from build123d import *

# Parameters (mm, degrees)
F0_W     = 99.991299
F0_H     = 51.749203
F1_DEPTH = 1
F2_R     = 3.884772
F3_DEPTH = 1.001
F4_R     = 2.651648
F5_DEPTH = 25.4


with BuildPart() as f1:
    # F0 (on Top) → F1 (new body)
    with BuildSketch(Plane.XY):
        with Locations((49.995649, 25.874601)):
            Rectangle(F0_W, F0_H)
    extrude(amount=F1_DEPTH)

    # F2 (on face) → F3 (cut, through all)
    with BuildSketch(Plane.XY.offset(1)):
        with Locations((73.43898, 21.35068)):
            Circle(F2_R)
    extrude(amount=-F3_DEPTH, mode=Mode.SUBTRACT)

    # F4 (on face) → F5 (join)
    with BuildSketch(Plane.XY.offset(1)):
        with Locations((28.457584, 20.000773)):
            Circle(F4_R)
    extrude(amount=F5_DEPTH)


solid = f1.part
Can you work these out from the model? Positions are in its coordinate system, mm. Coordinates: 2 decimals unless noted, no trailing zeros. Write each loop counter-clockwise with the first axis right and the second up, starting at its lowest first coordinate (ties: lowest second). Pieces come first, ordered by that corner, then holes. Notation, with made-up numbers: (39.5, 79.25) - (97.5, 79.25) arc R24 cw to (97.5, 110.25) - close; hole circle Ø3 at (29.5, 68.5). An arc over 180 degrees is marked (long way). Return JSON: item names as keys, results as strings. Group by question number.
Item 1: If we section it at C-C (x = 92): Write out the boundary of the cut face in (y, z), then the cut area to 3 significant figures.
Item 2: If we section it at B-B (x = 71.5): Write out the boundary of the cut face in (y, z), then the cut area to 3 significant figures.
Item 3: If we section it at D-D (y = 26.5): Write out the boundary of the cut face in (x, z), then the cut area to 4 significant figures.
Item 4: If we section it at A-A (y = 18.5): Write out the boundary of the cut face in (x, z).
Item 5: Please list where these lines run through material, in increasing order: probe 1 along Z at (x, y) = (22.5, 18.5); probe 2 along X at (y, z) = (20, 6).
Item 6: We'd pull the mould along X, two halves only. Please class faces 1 (the face through (77.144, 22.518, 0.507)), 2 (the face through (49, 26, 0)), 3 (the face through (26.35, 18.39, 13.52)): pulls with the +X half, pulls with the -X half, needs draft (parallel to the pull), parting line crosses it, or undercut.
Item 7: I'm going to push flat-ended pins straight in: pin 1 Ø1.5 at (x, y) = (54.5, 35.5) entering from +Z; pin 2 Ø12 at (y, z) = (31.5, 20) entering from -X. Where does each tip first touch, or does it pass through?
Return value:
{
 "1": {"outline": "(0, 0) - (51.75, 0) - (51.75, 1) - (0, 1) - close", "area": "51.7 mm^2"},
 "2": {"outline": "(0, 0) - (17.98, 0) - (17.98, 1) - (0, 1) - close; (24.72, 0) - (51.75, 0) - (51.75, 1) - (24.72, 1) - close", "area": "45.0 mm^2"},
 "3": {"outline": "(0, 0) - (99.99, 0) - (99.99, 1) - (0, 1) - close", "area": "100.0 mm^2"},
 "4": {"outline": "(0, 0) - (70.8, 0) - (70.8, 1) - (30.64, 1) - (30.64, 26.4) - (26.27, 26.4) - (26.27, 1) - (0, 1) - close; (76.08, 0) - (99.99, 0) - (99.99, 1) - (76.08, 1) - close"},
 "5": {"probe 1": "z = 0 to 1", "probe 2": "x = 25.81 to 31.11"},
 "6": {"face 1": "undercut", "face 2": "needs draft", "face 3": "parting line crosses it"},
 "7": {"pin 1": "stops at z = 1", "pin 2": "passes through"}
}
